Study the drawing (mm; zero at the part's minimum x, y, z) and answer. Round coordinates to 2 decimals unless told otherwise and drop trailing zeros. Order: outer loops, then holes, each group sorted by start corner. A loop starts at its lowest first (then second) coordinate and runs counter-clockwise, first axis right, second up. Notation, with made-up numbers: M -37.5,45 L -26.5,45 A30 ccw -26.5,77 Z; hole C 55.25,53.5 d4. An arc over 180 degrees is marked long. Put each result on its own line as item: value. Start each with the question number.
1. The part is cut by section B-B (z = 44.45). Give the vertices of the cut face in (x, y).
2. The mould has two halves that part along X. Classify the marked faces 1, 2, 3 and 4: +X half, -X half, draft (parallel to the pull), parting line (faces both ways), or undercut.
3. Each of these flat-tipped pins is pushed along its axis until it touches: pin 1 Ø3 at (y, z) = (1, 19) entering from -X; pin 2 Ø1.9 at (x, y) = (14, 3) entering from +Z; pin 3 Ø1.9 at (x, y) = (68, 3.5) entering from -Z. Where does it stop, or does it pass through?
4. Consider line 1 (X direction, y = 2.3, z = 44.45); line 2 (Z direction, x = 8.89, y = 0.75). Determine where each line is inside the solid, lowest interval first.
5. The part is cut by section D-D (z = 80.01). Give the vertices of the cut face in (x, y), then the cut area to 3 significant figures.
6. The part is cut by section C-C (y = 1.25). Count the separate pieces of the cut face and the enclosed holes in it, then the cut area to 3 significant figures.
7. The part is cut by section A-A (x = 44.45). Give the vertices of the cut face in (y, z), then the cut area to 3 significant figures.
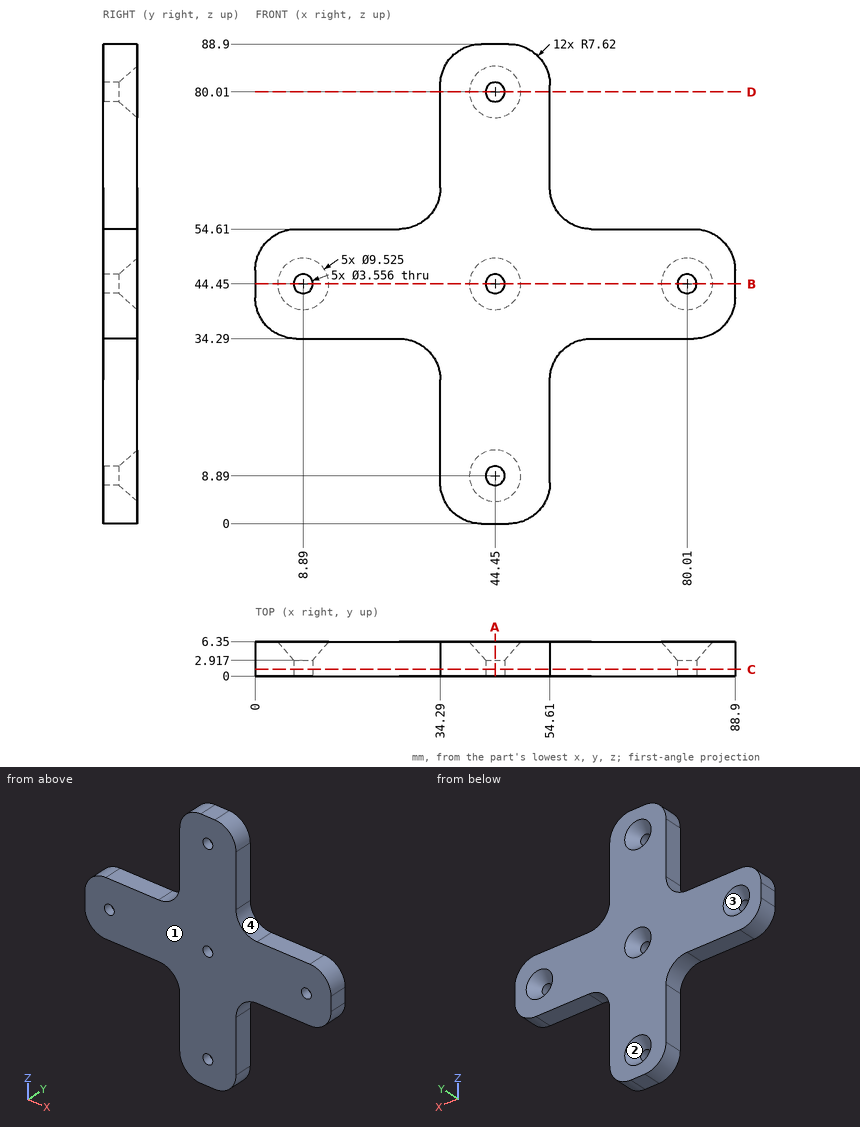
Resolved:
1. outline: M 0,0 L 7.11,0 L 7.11,2.92 L 4.13,6.35 L 0,6.35 Z; M 10.67,0 L 42.67,0 L 42.67,2.92 L 39.69,6.35 L 13.65,6.35 L 10.67,2.92 Z; M 46.23,0 L 78.23,0 L 78.23,2.92 L 75.25,6.35 L 49.21,6.35 L 46.23,2.92 Z; M 81.79,0 L 88.9,0 L 88.9,6.35 L 84.77,6.35 L 81.79,2.92 Z
2. face 1: draft
2. face 2: undercut
2. face 3: undercut
2. face 4: +X half
3. pin 1: x = 34.29
3. pin 2: z = 54.61
3. pin 3: z = 34.29
4. line 1: 0 to 7.11, 10.67 to 42.67, 46.23 to 78.23, 81.79 to 88.9
4. line 2: 34.29 to 42.67, 46.23 to 54.61
5. outline: M 34.29,0 L 42.67,0 L 42.67,2.92 L 39.69,6.35 L 34.29,6.35 Z; M 46.23,0 L 54.61,0 L 54.61,6.35 L 49.21,6.35 L 46.23,2.92 Z
5. area: 96.2 mm2
6. separate pieces: 1
6. enclosed holes: 5
6. area: 3,100 mm2
7. outline: M 0,0 L 6.35,0 L 6.35,4.13 L 2.92,7.11 L 0,7.11 Z; M 0,10.67 L 2.92,10.67 L 6.35,13.65 L 6.35,39.69 L 2.92,42.67 L 0,42.67 Z; M 0,46.23 L 2.92,46.23 L 6.35,49.21 L 6.35,75.25 L 2.92,78.23 L 0,78.23 Z; M 0,81.79 L 2.92,81.79 L 6.35,84.77 L 6.35,88.9 L 0,88.9 Z
7. area: 466 mm2
